Geometry check sheet. Reference: the model listing, model coordinates, mm. Coordinates: 2 decimals unless noted, no trailing zeros. Loops run counter-clockwise (first coordinate to the right, second up) from the corner with the lowest first, then second, coordinate; pieces in that order, holes last.
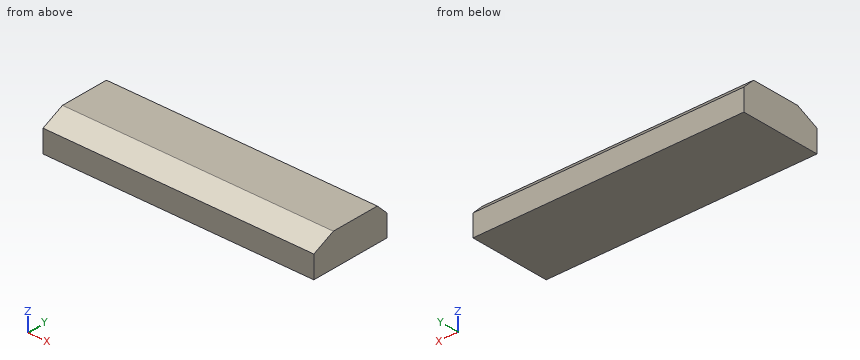
from build123d import *

# Parameters (mm, degrees)
SKETCH_1_W      = 25
SKETCH_1_H      = 7.5
EXTRUDE_1_DEPTH = 3
CHAMFER_1_SIZE  = 1
CHAMFER_2_SIZE  = 2
CHAMFER_2_SIZE2 = 0.932615316


with BuildPart() as part:
    # Эскиз1 → Вытянуть1 (new body)
    with BuildSketch(Plane.XY):
        with Locations((0, 0.25)):
            Rectangle(SKETCH_1_W, SKETCH_1_H)
    extrude(amount=EXTRUDE_1_DEPTH)

    # Фаска1
    chamfer_1_edges = [part.edges().sort_by_distance(p)[0] for p in [
        (0, 4, 3),
    ]]
    chamfer(chamfer_1_edges, length=CHAMFER_1_SIZE)

    # Фаска2
    chamfer_2_edges = [part.edges().sort_by_distance(p)[0] for p in [
        (0, -3.5, 3),
    ]]
    chamfer_2_side = [part.faces().sort_by_distance(p)[0] for p in [
        (0, -0.25, 3),
    ]]
    chamfer(chamfer_2_edges, length=CHAMFER_2_SIZE, length2=CHAMFER_2_SIZE2, reference=chamfer_2_side[0])


solid = part.part
(1) Scan lines: L1, parallel to Z at x = 8.75, y = 3.25; L2, parallel to Z at x = 10.25, y = -2.5; L3, parallel to Y at x = -11, z = 2.6. Record each from-to range of solid material in increasing order.
Findings:
L1: z = 0 to 2.75
L2: z = 0 to 2.53
L3: y = -2.36 to 3.4
(2) Sectioned sample at C-C on z = 2.75. Record the cut outline in (x, y), and give its area (3 significant figures).
Findings:
outline: (-12.5, -2.04) - (12.5, -2.04) - (12.5, 3.25) - (-12.5, 3.25) - close
area: 132 mm2
(3) Gauge pin test, flat end, axial feed: pin 1 Ø1.5 at (x, y) = (0.5, -1) entering from -Z. Record the tip position at first contact, or that the pin passes through.
Findings:
pin 1: stops at z = 0
(4) Sectioned sample at A-A on x = -7. Record the cut outline in (y, z), and give its area (3 significant figures).
Findings:
outline: (-3.5, 0) - (4, 0) - (4, 2) - (3, 3) - (-1.5, 3) - (-3.5, 2.07) - close
area: 21.1 mm2
(5) Sectioned sample at B-B on y = 3.75. Record the cut outline in (x, z), and give its area (4 significant figures).
Findings:
outline: (-12.5, 0) - (12.5, 0) - (12.5, 2.25) - (-12.5, 2.25) - close
area: 56.25 mm2
